Could you check a few things on this model? Use its own coordinates, in mm. A direction names the side the tool comes from. Round coordinates to 2 decimals unless told otherwise and drop trailing zeros. Write each loop counter-clockwise with the first axis right and the second up, starting at its lowest first coordinate (ties: lowest second). Pieces come first, ordered by that corner, then holes. Notation, with made-up numbers: M 80.5,63 L 132.5,63 A27 cw 132.5,87 Z; hole C 30.5,21.5 d1. An arc over 180 degrees is marked long. One line per item, written item: value. Start each with the question number.
(1) I'm going to push flat-ended pins straight in: pin 1 Ø13 at (x, y) = (72.5, 0) entering from -Z; pin 2 Ø18.5 at (x, z) = (-0.5, 34.5) entering from +Y; pin 3 Ø6 at (x, z) = (72.5, 51.5) entering from +Y. Where does each tip first touch, or does it pass through?
(2) Thinking about a two-plate mould opening in X: for faces 6 (the face through (39.464, 61.59, 0.133)), 7 (the face through (78, 0, 42.875)), 8 (the face through (-39.365, -61.689, -0.133)), which applies, released by +X, released by -X, zero draft, split by the parting line, or undercut?
(3) If I drill on L1, parallel to X at y = -40.5, z = -3.5 (3 decimals); L2, parallel to Z at x = -27.5, y = 26.5 (3 decimals); L3, parallel to Y at x = 24, z = 10, over which ranges is the centre line in solid material (lowest first)?
(4) I want a section at D-D on y = 35. Please give me the cut outline in (x, z) (3 decimals).
(5) I want a section at A-A on y = 20. Please give me the cut outline in (x, z) (3 decimals), and give its area (3 significant figures).
(6) I want a section at C-C on x = 7.5. Please give me the cut outline in (y, z) (1 decimal).
(7) Which directions (+Z, -Z, +X, -X, +Y, -Y) give clear straight access to the entire face, cutting with the end or side of a thin tool? Please do faces 1 (the face through (22.225, 17, 18)), 2 (the face through (22.225, -17, 18)), 3 (the face through (52, -25.4, 48)), 4 (the face through (52, 25.4, 48)), 5 (the face through (45.8, -0.4, 38.1)).
```python
from build123d import *

# Parameters (mm, degrees)
F1_DEPTH = 63.5
F2_DEPTH = 25.4
F3_DEPTH = 7.9375
F5_R     = 6.35


with BuildPart() as f1:
    # F0 (on Front) → F1 (new body, symmetric)
    with BuildSketch(Plane.XZ):
        Polygon((41.275, -9.525), (41.275, 9.525), (22.225, 9.525), (-41.275, 9.525), (-41.275, -9.525), align=None)
    extrude(amount=F1_DEPTH, both=True)

    # F0 (on Front) → F2 (join, symmetric)
    with BuildSketch(Plane.XZ):
        with BuildLine():
            Line((22.225, 9.525), (41.275, 9.525))
            Line((41.275, 9.525), (41.275, 27.0002))
            ThreePointArc((41.275, 27.0002), (45.9246798487, 38.2255201513), (57.15, 42.8752))
            Line((57.15, 42.8752), (60.325, 42.8752))
            Line((60.325, 42.8752), (60.325, 61.9252))
            Line((60.325, 61.9252), (57.15, 61.9252))
            Line((57.15, 61.9252), (28.1752493255, 46.4994166087))
            ThreePointArc((28.1752493255, 46.4994166087), (23.7456680032, 37.1936404813), (22.225, 27.0002))
            Line((22.225, 27.0002), (22.225, 9.525))
        make_face()
        Polygon((60.325, 61.9252), (60.325, 42.8752), (99.8372383581, 42.8752), (99.5686697629, 61.9252), align=None)
    extrude(amount=F2_DEPTH, both=True)

    # F0 (on Front) → F3 (join, symmetric)
    with BuildSketch(Plane.XZ):
        with BuildLine():
            Line((-41.275, 9.525), (22.225, 9.525))
            Line((22.225, 9.525), (22.225, 27.0002))
            ThreePointArc((22.225, 27.0002), (23.7456680032, 37.1936404813), (28.1752493255, 46.4994166087))
            Line((28.1752493255, 46.4994166087), (-41.275, 9.525))
        make_face()
    extrude(amount=F3_DEPTH, both=True)

    # F0 (on Front) → F4 (revolve)
    with BuildSketch(Plane.XZ):
        Polygon((99.5686697629, 61.9252), (99.8372383581, 42.8752), (99.9045595527, 38.1), (111.125, 38.1), (111.125, 66.675), (99.5017066598, 66.675), align=None)
    revolve(axis=Axis((99.7031331062, 0, 52.3875), (0.0140966882, 0, -0.9999006368)))

    # F5
    f5_edges = [f1.edges().sort_by_distance(p)[0] for p in [
        (41.275, -63.5, 0),
        (-41.275, -63.5, 0),
        (41.275, 63.5, 0),
        (-41.275, 63.5, 0),
    ]]
    fillet(f5_edges, radius=F5_R)


solid = f1.part
```
Found:
1. pin 1: stops at z = 42.88
1. pin 2: stops at y = 7.94
1. pin 3: stops at y = 25.4
2. face 6: released by +X
2. face 7: undercut
2. face 8: released by -X
3. L1: x = -41.275 to 41.275
3. L2: z = -9.525 to 9.525
3. L3: y = -25.4 to 25.4
4. outline: M -41.275,-9.525 L 41.275,-9.525 L 41.275,9.525 L -41.275,9.525 Z
5. outline: M -41.275,-9.525 L 41.275,-9.525 L 41.275,27 A15.875 cw 57.15,42.875 L 99.837,42.875 L 99.569,61.925 L 57.15,61.925 L 28.175,46.499 A34.925 ccw 22.225,27 L 22.225,9.525 L -41.275,9.525 Z
5. area: 3,390 mm²
6. outline: M -63.5,-9.5 L 63.5,-9.5 L 63.5,9.5 L 7.9,9.5 L 7.9,35.5 L -7.9,35.5 L -7.9,9.5 L -63.5,9.5 Z
7. face 1: +Z, -X, +Y
7. face 2: +Z, -X, -Y
7. face 3: +Z, +X, -X, -Y
7. face 4: +Z, +X, -X, +Y
7. face 5: -Z, +Y, -Y
